from build123d import *

# Parameters (mm, degrees)
F0_W     = 1.27
F0_H     = 5.7522215727
F0_W_2   = 6.1100403625
F0_H_2   = 1.27
F0_H_3   = 2.8992746613
F1_DEPTH = 12.7
F2_W     = 50.8
F2_H     = 25.4
F3_DEPTH = 2.54
F5_DEPTH = 50.8
F6_W     = 50.8
F6_H     = 25.4
F7_DEPTH = 0.254


with BuildPart() as f1:
    # F0 (on Top) → F1 (new body)
    with BuildSketch(Plane.XY):
        Polygon((27.4962335825, 5.3974989146), (-23.3037664175, 5.3974989146), (-23.3037664175, -20.0025010854), (0.6083042244, -20.0025010854), (0.6083042244, -18.7325010854), (-8.6501812091, -18.7325010854), (-9.9201812091, -18.7325010854), (-22.0337664175, -18.7325010854), (-22.0337664175, -4.8546069302), (-22.0337664175, -3.5846069302), (-22.0337664175, 4.1274989146), (-11.1901812091, 4.1274989146), (-9.9201812091, 4.1274989146), (3.0415252629, 4.1274989146), (3.0415252629, -1.2985680951), (4.3115252629, -1.2985680951), (4.3115252629, 4.1274989146), (26.2262335825, 4.1274989146), (26.2262335825, -4.8546069302), (26.2262335825, -6.1246069302), (26.2262335825, -18.7325010854), (9.3469638377, -18.7325010854), (9.3469638377, -20.0025010854), (27.4962335825, -20.0025010854), align=None)
        with Locations((-9.2851812091, -15.8563902991)):
            Rectangle(F0_W, F0_H)
        with Locations((23.1712134013, -5.4896069302)):
            Rectangle(F0_W_2, F0_H_2)
        with BuildLine():
            Line((-22.0337664175, -3.5846069302), (-22.0337664175, -4.8546069302))
            Line((-22.0337664175, -4.8546069302), (-11.1901812091, -4.8546069302))
            ThreePointArc((-11.1901812091, -4.8546069302), (-10.292155597, -5.2265813181), (-9.9201812091, -6.1246069302))
            Line((-9.9201812091, -6.1246069302), (-9.9201812091, -10.781369172))
            Line((-9.9201812091, -10.781369172), (-8.6501812091, -10.781369172))
            Line((-8.6501812091, -10.781369172), (-8.6501812091, -6.1246069302))
            Line((-8.6501812091, -6.1246069302), (16.8178286403, -6.1246069302))
            Line((16.8178286403, -6.1246069302), (16.8178286403, -4.8546069302))
            Line((16.8178286403, -4.8546069302), (4.3115252629, -4.8546069302))
            Line((4.3115252629, -4.8546069302), (4.3115252629, -2.6728871744))
            Line((4.3115252629, -2.6728871744), (3.0415252629, -2.6728871744))
            Line((3.0415252629, -2.6728871744), (3.0415252629, -4.8546069302))
            Line((3.0415252629, -4.8546069302), (-8.6501812091, -4.8546069302))
            ThreePointArc((-8.6501812091, -4.8546069302), (-9.5482068213, -4.4826325423), (-9.9201812091, -3.5846069302))
            Line((-9.9201812091, -3.5846069302), (-9.9201812091, -0.5181303131))
            Line((-9.9201812091, -0.5181303131), (-11.1901812091, -0.5181303131))
            Line((-11.1901812091, -0.5181303131), (-11.1901812091, -3.5846069302))
            Line((-11.1901812091, -3.5846069302), (-22.0337664175, -3.5846069302))
        make_face()
        with Locations((-10.5551812091, 2.6778615839)):
            Rectangle(F0_W, F0_H_3)
    extrude(amount=F1_DEPTH)

    # F2 (on face) → F3 (join)
    with BuildSketch(Plane.XY.offset(12.7)):
        with Locations((2.0962335825, -7.3025010854)):
            Rectangle(F2_W, F2_H)
    extrude(amount=F3_DEPTH)

    # F4 (on face) → F5 (join)
    with BuildSketch(Plane(origin=(-23.3037664175, 0, 0), x_dir=(0, -1, 0), z_dir=(-1, 0, 0))):
        Polygon((7.3025010854, 24.7875675559), (-5.3974989146, 15.24), (20.0025010854, 15.24), align=None)
    extrude(amount=-F5_DEPTH)

    # F6 (on face) → F7 (join)
    with BuildSketch(Plane(origin=(0, 0, 0), x_dir=(1, 0, 0), z_dir=(0, 0, -1))):
        with Locations((2.0962335825, 7.3025010854)):
            Rectangle(F6_W, F6_H)
    extrude(amount=F7_DEPTH)


solid = f1.part
Read the model definition and answer for the solid it produces. Units are mm, in the model's axes. A direction names the side the tool comes from. Coordinates: 2 decimals unless noted, no trailing zeros. Loops run counter-clockwise (first coordinate to the right, second up) from the corner with the lowest first, then second, coordinate; pieces in that order, holes last. Notation, with made-up numbers: (43.5, 53) -> (91.5, 53) arc R21 ccw to (91.5, 64) -> close; hole circle Ø1 at (14, 89.5). An arc over 180 degrees is marked (long way). Write item = value, one per line. Start each with the question number.
1) The part is cut by section D-D, the plane z = 21.5. Determine the outline of the cut face in (x, y).
2) The mould has two halves that part along Z. Classify faces 1 (the face through (27.496, -7, 10)), 2 (the face through (-9.92, -8, 6)): pulls with the +Z half, pulls with the -Z half, needs draft (parallel to the pull), parting line crosses it, or undercut.
3) Find the intervals of material crossed by L1, parallel to X at y = -14.75, z = 6.5; L2, parallel to X at y = -2.25, z = 8.5; L3, parallel to Y at x = 24, z = 9.5, in increasing order. Write a range as from..to.
4) The part is cut by section C-C, the plane y = -2. Determine the outline of the cut face in (x, z), plus the area to 3 significant figures.
5) For faces 3 (the face through (9.347, -19, 6)), 4 (the face through (-11.19, 3, 6)), 5 (the face through (-23.304, -7, 10)), determine the directions among +Z, -Z, +X, -X, +Y, -Y from which every point of the face is accessible in a straight line to the end or side of a thin tool.
6) The part is cut by section A-A, the plane x = 6. Determine the outline of the cut face in (y, z).
7) Given P1, Ø5, axis at x = 14, y = -3.5, coming from the +Z side; P2, Ø10, axis at x = -18, z = 21.5, coming from the +Y side; P3, Ø2, axis at x = -12, z = 17.5, coming from the -Y side, each flat-ended and moving along its own axis, determine where each tip first touches the part or whether it passes through.
8) The part is cut by section B-B, the plane x = -1. Determine the outline of the cut face in (y, z), plus the area to 3 significant figures.
Result:
q1.outline = (-23.3, -11.68) -> (27.5, -11.68) -> (27.5, -2.93) -> (-23.3, -2.93) -> close
q2.face_1 = needs draft
q2.face_2 = undercut
q3.L1 = -23.3..-22.03, -9.92..-8.65, 26.23..27.5
q3.L2 = -23.3..-22.03, -11.19..-9.92, 26.23..27.5
q3.L3 = -20..-18.73, -6.12..-4.85, 4.13..5.4
q4.outline = (-23.3, -0.25) -> (27.5, -0.25) -> (27.5, 20.8) -> (-23.3, 20.8) -> close; hole (-22.03, 0) -> (-11.19, 0) -> (-11.19, 12.7) -> (-22.03, 12.7) -> close; hole (-9.92, 0) -> (26.23, 0) -> (26.23, 12.7) -> (-9.92, 12.7) -> close
q4.area = 473 mm²
q5.face_3 = -Y
q5.face_4 = none
q5.face_5 = +Z, -Z, -X, +Y, -Y
q6.outline = (-20, -0.25) -> (5.4, -0.25) -> (5.4, 15.24) -> (-7.3, 24.79) -> (-20, 15.24) -> (-20, 12.7) -> (-6.12, 12.7) -> (-6.12, 0) -> (-20, 0) -> close; hole (-4.85, 0) -> (4.13, 0) -> (4.13, 12.7) -> (-4.85, 12.7) -> close
q7.P1 = 23.81
q7.P2 = 3.72
q7.P3 = -18.33
q8.outline = (-20, -0.25) -> (5.4, -0.25) -> (5.4, 15.24) -> (-7.3, 24.79) -> (-20, 15.24) -> close; hole (-18.73, 0) -> (-6.12, 0) -> (-6.12, 12.7) -> (-18.73, 12.7) -> close; hole (-4.85, 0) -> (4.13, 0) -> (4.13, 12.7) -> (-4.85, 12.7) -> close
q8.area = 241 mm²
